Source: three-view drawing plus pictorial views. Frame: mm from the lowest corner of the part. A direction names the side the tool comes from. Round coordinates to 2 decimals unless told otherwise and drop trailing zeros. Order: outer loops, then holes, each group sorted by start corner. A loop starts at its lowest first (then second) coordinate and runs counter-clockwise, first axis right, second up. Notation, with made-up numbers: (37, 81.5) -> (77, 81.5) arc R16 ccw to (77, 107.5) -> close; hole circle Ø2 at (76.25, -15.5). An arc over 180 degrees is marked (long way). Use a Markdown table: item, result.
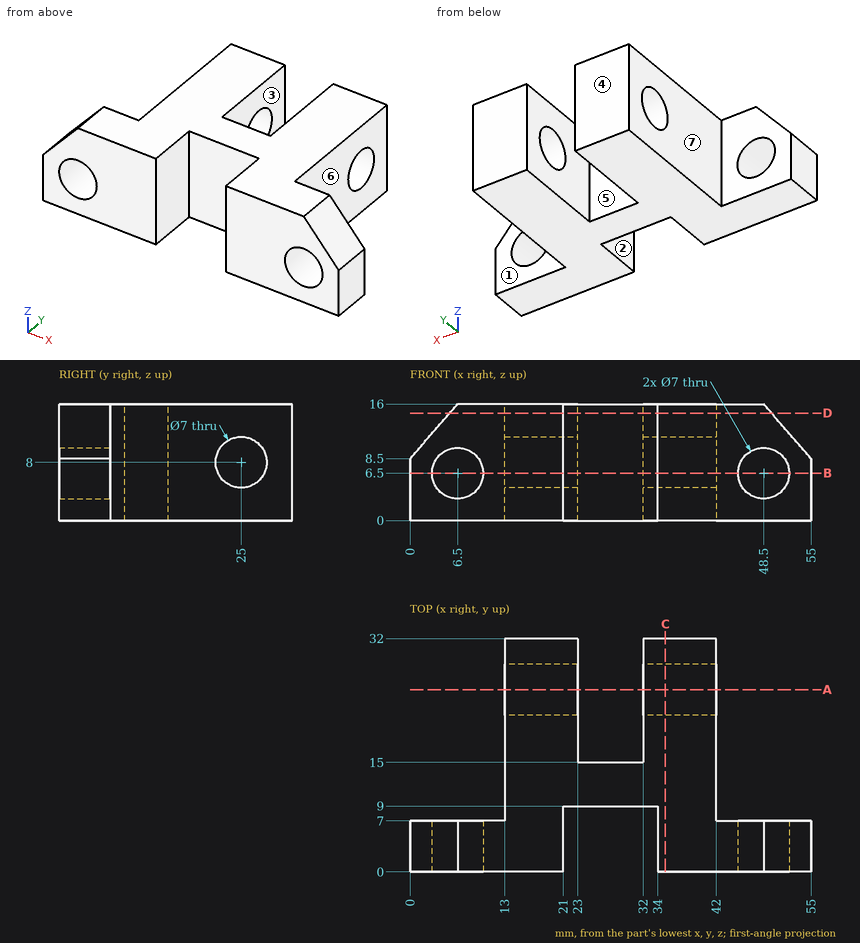
1) Cut plane B-B on z = 6.5. Count the separate pieces of the cut face and the enclosed holes in it, and give its area (3 significant figures).
Results found:
| item | result |
|---|---|
| separate pieces | 5 |
| enclosed holes | 0 |
| area | 616 mm² |
2) Cut plane A-A on y = 25. Return loops of the section in (x, z), and give its area (3 significant figures).
Results found:
| item | result |
|---|---|
| outline | (13, 0) -> (23, 0) -> (23, 4.5) -> (13, 4.5) -> close; (13, 11.5) -> (23, 11.5) -> (23, 16) -> (13, 16) -> close; (32, 0) -> (42, 0) -> (42, 4.5) -> (32, 4.5) -> close; (32, 11.5) -> (42, 11.5) -> (42, 16) -> (32, 16) -> close |
| area | 180 mm² |
3) Pin query (flat end, axial travel): pin 1 Ø9 at (y, z) = (25, 8) entering from -X; pin 2 Ø6.5 at (x, z) = (6.5, 6.5) entering from -Y; pin 3 Ø5 at (y, z) = (13.5, 8) entering from +X. Return the tip coordinate at first contact, or that it passes through.
Results found:
| item | result |
|---|---|
| pin 1 | stops at x = 13 |
| pin 2 | passes through |
| pin 3 | stops at x = 42 |
4) Line query: L1, parallel to X at y = 29.5, z = 4.5; L2, parallel to Y at x = 40, z = 7.75; L3, parallel to X at y = 3.5, z = 6.5. Output: solid intervals per line, ascending. Write a range as [from, to].
Results found:
| item | result |
|---|---|
| L1 | x = [13, 23], [32, 42] |
| L2 | y = [0, 21.51], [28.49, 32] |
| L3 | x = [0, 3], [10, 21], [34, 45], [52, 55] |
5) Cut plane C-C on x = 35. Return loops of the section in (y, z), and give its area (3 significant figures).
Results found:
| item | result |
|---|---|
| outline | (0, 0) -> (32, 0) -> (32, 16) -> (0, 16) -> close; hole circle Ø7 at (25, 8) |
| area | 474 mm² |
6) Cut plane D-D on z = 14.75. Return loops of the section in (x, y).
Results found:
| item | result |
|---|---|
| outline | (5.42, 0) -> (21, 0) -> (21, 9) -> (34, 9) -> (34, 0) -> (49.58, 0) -> (49.58, 7) -> (42, 7) -> (42, 32) -> (32, 32) -> (32, 15) -> (23, 15) -> (23, 32) -> (13, 32) -> (13, 7) -> (5.42, 7) -> close |
7) Pull-direction query (X, two-part tool) for the marked faces 4, 5, 6 and 7; classes: +X half, -X half, draft (parallel to the pull), parting line (faces both ways), or undercut.
Results found:
| item | result |
|---|---|
| face 4 | draft |
| face 5 | undercut |
| face 6 | +X half |
| face 7 | -X half |
8) Set-up query: the marked faces 1, 2 and 3. Return all of +Z, -Z, +X, -X, +Y, -Y with unobstructed straight access to the full face (end or side cutting, diameter ignored); none if empty.
Results found:
| item | result |
|---|---|
| face 1 | +Z, -Z, +X, +Y |
| face 2 | +Z, -Z, -Y |
| face 3 | +Z, -Z, +Y |
